Input: part model. Units: mm. Frame: model coordinates. A direction names the side the tool comes from. Coordinates: 2 decimals unless noted, no trailing zeros. Order: outer loops, then holes, each group sorted by start corner. A loop starts at its lowest first (then second) coordinate and runs counter-clockwise, first axis right, second up. Notation, with made-up numbers: (39, 14.25) - (63, 14.25) arc R18 ccw to (63, 42.25) - close; hole circle Ø5 at (47, -22). An arc over 180 degrees is marked (long way). Answer as CSV lines item,"result". Start each with the question number.
Item 1: Section B-B (x = 64.5). Output: boundary loops of the cut face in (y, z).
Item 2: First-contact query: pin 1 (12 mm diameter, centred on x = 43.5, y = 24.5, fed in from -Z); pin 2 (4 mm diameter, centred on x = 4, y = 32, fed in from -Z); pin 3 (1 mm diameter, centred on x = 5, y = -32, fed in from -Z). Flat tips, straight axial feed; report the tip coordinate or a pass-through.
Item 3: Access query for faces 1 (the flat face through (68, 33, 0)), 2 (the flat face through (11.609, 31, 1)), 3 (the flat face through (70, -34.25, 2)), 4 (the flat face through (10, 35, 2)), 5 (the flat face through (10, -35, 1)). Directions: +Z, -Z, +X, -X, +Y, -Y. A direction counts if a zero-diameter tool reaches every point of the face in a straight line with its end or side. Return the directions, or none.
Item 4: Section A-A (y = -3). Output: boundary loops of the cut face in (x, z), and give its area (3 significant figures).
Item 5: Section D-D (y = 19). Output: boundary loops of the cut face in (x, z), and give its area (3 significant figures).
Item 6: Material intervals for line 1 along X through (y, z) = (31, 3.15); line 2 along Y through (x, z) = (4.5, 2.55); line 3 along Y through (x, z) = (8.5, 1.5), sorted ascending.
Item 7: Draft query along Y for faces 6 (the flat face through (68.709, -33, 2)), 7 (the flat face through (75, 1, 4)), 8 (the flat face through (38, 37.5, 4)). Return one class per face: +Y half, -Y half, draft (parallel to the pull), parting line (faces both ways), or undercut.
from build123d import *

# Parameters (mm, degrees)
RESSALTO_EXTRUS_O1_DEPTH   = 3
RESSALTO_EXTRUS_O1_2_DEPTH = 3
RESSALTO_EXTRUS_O1_3_DEPTH = 3
RESSALTO_EXTRUS_O1_4_DEPTH = 3
RESSALTO_EXTRUS_O2_DEPTH   = 2
ESBO_O13_W                 = 0.999795876
ESBO_O13_H                 = 5.679795897
RESSALTO_EXTRUS_O3_DEPTH   = 3
CORTE_EXTRUS_O4_DEPTH      = 3
ESBO_O22_W                 = 3
ESBO_O22_H                 = 2.1
ESBO_O22_H_2               = 8
RESSALTO_EXTRUS_O5_DEPTH   = 4
ESBO_O15_W                 = 3.5
ESBO_O15_H                 = 3.5
CORTE_EXTRUS_O1_DEPTH      = 3.5
ESBO_O16_W                 = 8
ESBO_O16_H                 = 8
CORTE_EXTRUS_O2_DEPTH      = 1
ESBO_O18_W                 = 7
ESBO_O18_H                 = 5
CORTE_EXTRUS_O3_DEPTH      = 10


with BuildPart() as part:
    # Esbo_o1 → Ressalto-extrus_o1 (new body)
    with BuildSketch(Plane.XY):
        with BuildLine():
            Line((10, -36.5), (10, -31.8))
            ThreePointArc((10, -31.8), (9.707106781, -31.092893219), (9, -30.8))
            Line((9, -30.8), (8.409000397, -30.8))
            Line((8.409000397, -30.8), (8.409000397, -27.5))
            Line((8.409000397, -27.5), (0, -27.5))
            Line((0, -27.5), (0, -36.5))
            ThreePointArc((0, -36.5), (0.292893219, -37.207106781), (1, -37.5))
            Line((1, -37.5), (9, -37.5))
            ThreePointArc((9, -37.5), (9.707106781, -37.207106781), (10, -36.5))
        make_face()
    extrude(amount=RESSALTO_EXTRUS_O1_DEPTH)



with BuildPart() as body_2:
    # Esbo_o1 → Ressalto-extrus_o1 2 (new body)
    with BuildSketch(Plane.XY):
        with BuildLine():
            Line((75, -36.5), (75, -28.5))
            ThreePointArc((75, -28.5), (74.707106781, -27.792893219), (74, -27.5))
            Line((74, -27.5), (66.909000397, -27.5))
            ThreePointArc((66.909000397, -27.5), (66.201893616, -27.792893219), (65.909000397, -28.5))
            Line((65.909000397, -28.5), (65.909000397, -36.5))
            ThreePointArc((65.909000397, -36.5), (66.201893616, -37.207106781), (66.909000397, -37.5))
            Line((66.909000397, -37.5), (74, -37.5))
            ThreePointArc((74, -37.5), (74.707106781, -37.207106781), (75, -36.5))
        make_face()
    extrude(amount=RESSALTO_EXTRUS_O1_2_DEPTH)


with BuildPart() as body_3:
    # Esbo_o1 → Ressalto-extrus_o1 3 (new body)
    with BuildSketch(Plane.XY):
        with BuildLine():
            Line((65.909000397, 36.5), (65.909000397, 28.5))
            ThreePointArc((65.909000397, 28.5), (66.201893616, 27.792893219), (66.909000397, 27.5))
            Line((66.909000397, 27.5), (75, 27.5))
            Line((75, 27.5), (75, 36.5))
            ThreePointArc((75, 36.5), (74.707106781, 37.207106781), (74, 37.5))
            Line((74, 37.5), (66.909000397, 37.5))
            ThreePointArc((66.909000397, 37.5), (66.201893616, 37.207106781), (65.909000397, 36.5))
        make_face()
    extrude(amount=RESSALTO_EXTRUS_O1_3_DEPTH)


with BuildPart() as body_4:
    # Esbo_o1 → Ressalto-extrus_o1 4 (new body)
    with BuildSketch(Plane.XY):
        with BuildLine():
            Line((9, 37.5), (1, 37.5))
            ThreePointArc((1, 37.5), (0.292893219, 37.207106781), (0, 36.5))
            Line((0, 36.5), (0, 28.5))
            ThreePointArc((0, 28.5), (0.292893219, 27.792893219), (1, 27.5))
            Line((1, 27.5), (7.409000397, 27.5))
            ThreePointArc((7.409000397, 27.5), (8.116107178, 27.792893219), (8.409000397, 28.5))
            Line((8.409000397, 28.5), (8.409000397, 30.8))
            Line((8.409000397, 30.8), (9, 30.8))
            ThreePointArc((9, 30.8), (9.71421429, 31.100072898), (9.999795876, 31.820204103))
            Line((9.999795876, 31.820204103), (9, 31.820204103))
            Line((9, 31.820204103), (9, 37.5))
        make_face()
    extrude(amount=RESSALTO_EXTRUS_O1_4_DEPTH)


with BuildPart() as part_1:
    add(part.part)

    add(body_2.part)  # Ressalto-extrus_o2 merges body 2

    add(body_3.part)  # Ressalto-extrus_o2 merges body 3

    add(body_4.part)  # Ressalto-extrus_o2 merges body 4
    # Esbo_o2 → Ressalto-extrus_o2 (add)
    with BuildSketch(Plane.XY.offset(3)):
        with BuildLine():
            Line((1, 37.5), (74, 37.5))
            ThreePointArc((74, 37.5), (74.707106781, 37.207106781), (75, 36.5))
            Line((75, 36.5), (75, -36.5))
            ThreePointArc((75, -36.5), (74.707106781, -37.207106781), (74, -37.5))
            Line((74, -37.5), (1, -37.5))
            ThreePointArc((1, -37.5), (0.292893219, -37.207106781), (0, -36.5))
            Line((0, -36.5), (0, 36.5))
            ThreePointArc((0, 36.5), (0.292893219, 37.207106781), (1, 37.5))
        make_face()
    extrude(amount=RESSALTO_EXTRUS_O2_DEPTH)

    # Esbo_o13 → Ressalto-extrus_o3 (add)
    with BuildSketch(Plane(origin=(0, 0, 3), x_dir=(-1, 0, 0), z_dir=(0, 0, -1))):
        with Locations((-9.499897938, 34.660102052)):
            Rectangle(ESBO_O13_W, ESBO_O13_H)
    extrude(amount=RESSALTO_EXTRUS_O3_DEPTH)

    # Esbo_o20 → Corte-extrus_o4 (cut)
    with BuildSketch(Plane(origin=(0, 0, 0), x_dir=(-1, 0, 0), z_dir=(0, 0, -1))):
        with BuildLine():
            Line((-8.409000397, 31.8), (-8.999795876, 31.8))
            ThreePointArc((-8.999795876, 31.8), (-9.706902657, 32.092893219), (-9.999795876, 32.8))
            Line((-9.999795876, 32.8), (-9.999795876, 30.8))
            Line((-9.999795876, 30.8), (-8.409000397, 30.8))
            Line((-8.409000397, 30.8), (-8.409000397, 31.8))
        make_face()
        with BuildLine():
            Line((-8.409000397, -30.8), (-8.409000397, -31.8))
            Line((-8.409000397, -31.8), (-9, -31.8))
            ThreePointArc((-9, -31.8), (-9.707106781, -32.092893219), (-10, -32.8))
            Line((-10, -32.8), (-10, -30.8))
            Line((-10, -30.8), (-8.409000397, -30.8))
        make_face()
    extrude(amount=-CORTE_EXTRUS_O4_DEPTH, mode=Mode.SUBTRACT)

    # Esbo_o22 → Ressalto-extrus_o5 (add)
    with BuildSketch(Plane(origin=(0, 0, 3), x_dir=(-1, 0, 0), z_dir=(0, 0, -1))):
        with Locations((-10.109000397, 30.55)):
            Rectangle(ESBO_O22_W, ESBO_O22_H)
        with Locations((-10.109000397, -30.55)):
            Rectangle(ESBO_O22_W, ESBO_O22_H)
        with Locations((-64.209000397, 32.5)):
            Rectangle(ESBO_O22_W, ESBO_O22_H_2)
        with Locations((-64.209000397, -32.5)):
            Rectangle(ESBO_O22_W, ESBO_O22_H_2)
    extrude(amount=RESSALTO_EXTRUS_O5_DEPTH)

    # Esbo_o15 → Corte-extrus_o1 (cut)
    with BuildSketch(Plane(origin=(0, 0, 0), x_dir=(-1, 0, 0), z_dir=(0, 0, -1))):
        with Locations((-4.25, -32.5)):
            Rectangle(ESBO_O15_W, ESBO_O15_H)
        with Locations((-4.25, 32.5)):
            Rectangle(ESBO_O15_W, ESBO_O15_H)
        with Locations((-70.459000397, 32.5)):
            Rectangle(ESBO_O15_W, ESBO_O15_H)
        with Locations((-70.459000397, -32.5)):
            Rectangle(ESBO_O15_W, ESBO_O15_H)
    extrude(amount=-CORTE_EXTRUS_O1_DEPTH, mode=Mode.SUBTRACT)

    # Esbo_o16 → Corte-extrus_o2 (cut)
    with BuildSketch(Plane(origin=(0, 0, 3), x_dir=(-1, 0, 0), z_dir=(0, 0, -1))):
        with Locations((-25.263712601, 2.900523079)):
            Rectangle(ESBO_O16_W, ESBO_O16_H)
    extrude(amount=-CORTE_EXTRUS_O2_DEPTH, mode=Mode.SUBTRACT)

    # Esbo_o18 → Corte-extrus_o3 (cut)
    with BuildSketch(Plane(origin=(0, 0, 3), x_dir=(-1, 0, 0), z_dir=(0, 0, -1))):
        with Locations((-25.3, -3)):
            Rectangle(ESBO_O18_W, ESBO_O18_H)
    extrude(amount=-CORTE_EXTRUS_O3_DEPTH, mode=Mode.SUBTRACT)


solid = part_1.part
Determined:
1,outline,"(-37.5, 3) - (-36.5, 3) - (-36.5, -1) - (-28.5, -1) - (-28.5, 3) - (28.5, 3) - (28.5, -1) - (36.5, -1) - (36.5, 3) - (37.5, 3) - (37.5, 5) - (-37.5, 5) - close"
2,pin 1,"stops at z = 3"
2,pin 2,"stops at z = 0"
2,pin 3,"stops at z = 3.5"
3,face 1,"-Z, +X, +Y, -Y"
3,face 2,"-Z, +Y, -Y"
3,face 3,"-Z"
3,face 4,"-Z, +Y"
3,face 5,"-Z, -Y"
4,outline,"(0, 3) - (21.8, 3) - (21.8, 5) - (0, 5) - close; (28.8, 3) - (75, 3) - (75, 5) - (28.8, 5) - close"
4,area,"136 mm^2"
5,outline,"(0, 3) - (75, 3) - (75, 5) - (0, 5) - close"
5,area,"150 mm^2"
6,line 1,"x = 0 to 2.5, 6 to 68.71, 72.21 to 75"
6,line 2,"y = -37.5 to -34.25, -30.75 to -27.5, 27.5 to 30.75, 34.25 to 37.5"
6,line 3,"y = -37.5 to -31.8, 31.8 to 37.5"
7,face 6,"undercut"
7,face 7,"draft"
7,face 8,"+Y half"
